The listing builds one solid part. Answer for the finished solid, in the listing's coordinates (mm). Face numbers are marked on the shaded views. A direction names the side the tool comes from. Round coordinates to 2 decimals unless told otherwise and drop trailing zeros. Loops run counter-clockwise (first coordinate to the right, second up) from the corner with the lowest first, then second, coordinate; pieces in that order, holes last. Notation, with made-up numbers: (25, 83) - (60, 83) arc R23 ccw to (60, 118) - close; hole circle Ø3 at (72.5, -0.75). An arc over 180 degrees is marked (long way). Write item = value, one per line. Start each with the question number.
1) Section D-D, the plane z = 16 is taken. Determine the outline of the cut face in (x, y), and give its area (3 significant figures).
2) A tool of negligible diameter and unlimited length cuts with its end or side. For the marked faces 5, 6 and 7, from which of +Z, -Z, +X, -X, +Y, -Y can it reach the whole face along a straight path? Write none if from no direction.
3) Section A-A, the plane z = 2 is taken. Determine the outline of the cut face in (x, y), and give its area (3 significant figures).
4) For a pull along X with two mould halves and no side action, classify the marked faces 1, 2, 3 and 4 as released by +X, released by -X, zero draft, split by the parting line, or undercut.
5) Section C-C, the plane y = 4 is taken. Determine the outline of the cut face in (x, z), and give its area (3 significant figures).
6) Section B-B, the plane x = 23.5 is taken. Determine the outline of the cut face in (y, z), and give its area (3 significant figures).
7) Straight lines are drawn through the part: line 1 along Z through (x, y) = (5, 5); line 2 along X through (y, z) = (0.5, 13); line 3 along Z through (x, y) = (-18, 3.25). For each, find the intervals that lie inside material, in ascending order.
from build123d import *

# Parameters (mm, degrees)
SKETCH1_W           = 50
SKETCH1_H           = 17.5
BOSS_EXTRUDE1_DEPTH = 7.5


with BuildPart() as part:
    # Sketch1 → Boss-Extrude1 (new body)
    with BuildSketch(Plane(origin=(0, 0, 0), x_dir=(1, 0, 0), z_dir=(0, 1, 0))):
        with BuildLine():
            Line((15, -20), (15, -12.4))
            Line((15, -12.4), (30, -12.4))
            Line((30, -12.4), (30, -20))
            Line((30, -20), (35, -20))
            ThreePointArc((35, -20), (38.535533906, -18.535533906), (40, -15))
            Line((40, -15), (40, 15))
            ThreePointArc((40, 15), (38.535533906, 18.535533906), (35, 20))
            Line((35, 20), (-35, 20))
            ThreePointArc((-35, 20), (-38.535533906, 18.535533906), (-40, 15))
            Line((-40, 15), (-40, -15))
            ThreePointArc((-40, -15), (-38.535533906, -18.535533906), (-35, -20))
            Line((-35, -20), (-30, -20))
            Line((-30, -20), (-30, -12.4))
            Line((-30, -12.4), (-15, -12.4))
            Line((-15, -12.4), (-15, -20))
            Line((-15, -20), (15, -20))
        make_face()
        with Locations((0, 1.25)):
            Rectangle(SKETCH1_W, SKETCH1_H, mode=Mode.SUBTRACT)
    extrude(amount=BOSS_EXTRUDE1_DEPTH)


solid = part.part
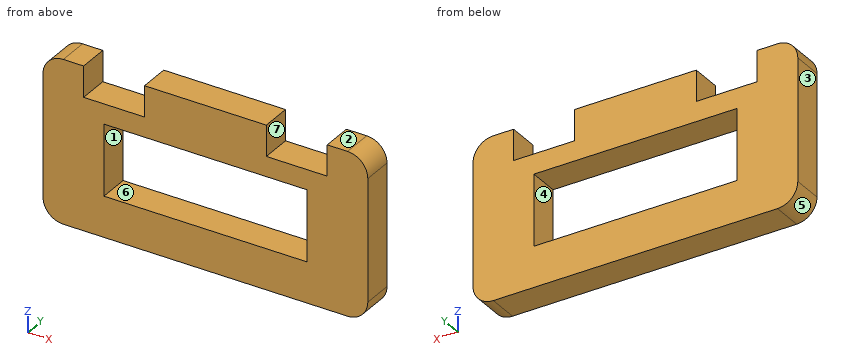
Geometry check:
q1.outline = (-39.9, 0) - (-30, 0) - (-30, 7.5) - (-39.9, 7.5) - close; (-15, 0) - (15, 0) - (15, 7.5) - (-15, 7.5) - close; (30, 0) - (39.9, 0) - (39.9, 7.5) - (30, 7.5) - close
q1.area = 373 mm2
q2.face_5 = -Z, -X, +Y, -Y
q2.face_6 = +Y, -Y
q2.face_7 = +Z, +Y, -Y
q3.outline = (-40, 0) - (-25, 0) - (-25, 7.5) - (-40, 7.5) - close; (25, 0) - (40, 0) - (40, 7.5) - (25, 7.5) - close
q3.area = 225 mm2
q4.face_1 = undercut
q4.face_2 = zero draft
q4.face_3 = released by -X
q4.face_4 = undercut
q5.outline = (-40, -15) arc R5 ccw to (-35, -20) - (35, -20) arc R5 ccw to (40, -15) - (40, 15) arc R5 ccw to (35, 20) - (30, 20) - (30, 12.4) - (15, 12.4) - (15, 20) - (-15, 20) - (-15, 12.4) - (-30, 12.4) - (-30, 20) - (-35, 20) arc R5 ccw to (-40, 15) - close; hole (-25, -10) - (25, -10) - (25, 7.5) - (-25, 7.5) - close
q5.area = 2,080 mm2
q6.outline = (0, -20) - (7.5, -20) - (7.5, -10) - (0, -10) - close; (0, 7.5) - (7.5, 7.5) - (7.5, 12.4) - (0, 12.4) - close
q6.area = 112 mm2
q7.line_1 = -20 to -10, 7.5 to 20
q7.line_2 = -40 to -30, -15 to 15, 30 to 40
q7.line_3 = -20 to -10, 7.5 to 12.4
